```python
from build123d import *

# Parameters (mm, degrees)
F1_DEPTH  = 160
F2_R      = 2.25
F3_DEPTH  = 16.001
F4_SIZE2  = 1
F4_SIZE   = 5
F5_SIZE2  = 5
F5_SIZE   = 1
F7_DEPTH  = 5
F8_R      = 2.25
F9_DEPTH  = 2
F10_SIZE  = 1.5
F11_SIZE  = 1
F12_W     = 12
F12_H     = 6
F12_W_2   = 4
F12_H_2   = 14
F13_DEPTH = 1


# Not quite as in the source:
# - a feature names something its author has since deleted; it is built from what else it names


with BuildPart() as f1:
    # F0 (on Front) → F1 (new body)
    with BuildSketch(Plane.XZ):
        Polygon((0, 16), (0, 0), (26.5, 0), (26.5, 16), (23.5, 16), (23.5, 6), (3, 6), (3, 16), align=None)
    extrude(amount=F1_DEPTH)

    # F2 (on face) → F3 (cut, through all)
    with BuildSketch(Plane(origin=(0, 0, 0), x_dir=(1, 0, 0), z_dir=(0, 0, -1))):
        with Locations((13.25, 146)):
            Circle(F2_R)
    extrude(amount=-F3_DEPTH, mode=Mode.SUBTRACT)

    # F4
    f4_edges = [f1.edges().sort_by_distance(p)[0] for p in [
        (23.5, -80, 16),
    ]]
    f4_side = f1.faces().sort_by_distance((23.5, -80, 11))[0]
    chamfer(f4_edges, length=F4_SIZE, length2=F4_SIZE2, reference=f4_side)

    # F5
    f5_edges = [f1.edges().sort_by_distance(p)[0] for p in [
        (3, -80, 16),
    ]]
    f5_side = f1.faces().sort_by_distance((1.5, -80, 16))[0]
    chamfer(f5_edges, length=F5_SIZE, length2=F5_SIZE2, reference=f5_side)

    # F6 (on face) → F7 (cut)
    with BuildSketch(Plane(origin=(0, 0, 0), x_dir=(1, 0, 0), z_dir=(0, 0, -1))):
        Polygon((15.2707259422, 149.5), (11.2292740578, 149.5), (9.2085481157, 146), (11.2292740578, 142.5), (15.2707259422, 142.5), (17.2914518843, 146), align=None)
    extrude(amount=-F7_DEPTH, mode=Mode.SUBTRACT)

    # F8 (on face) → F9 (join)
    with BuildSketch(Plane(origin=(0, 0, 0), x_dir=(1, 0, 0), z_dir=(0, 0, -1))):
        Polygon((15.2707259422, 149.5), (11.2292740578, 149.5), (9.2085481157, 146), (11.2292740578, 142.5), (15.2707259422, 142.5), (17.2914518843, 146), align=None)
        with Locations((13.25, 146)):
            Circle(F8_R, mode=Mode.SUBTRACT)
    extrude(amount=-F9_DEPTH)

    # F10
    f10_edges = [f1.edges().sort_by_distance(p)[0] for p in [
        (11, -146, 0),
    ]]
    chamfer(f10_edges, length=F10_SIZE)

    # F11
    f11_edges = [f1.edges().sort_by_distance(p)[0] for p in [
        (0, -80, 0),
        (13.25, 0, 0),
        (26.5, -80, 0),
        (13.25, -160, 0),
        (0, 0, 8),
        (26.5, 0, 8),
        (0, -160, 8),
        (26.5, -160, 8),
        (26.5, -80, 16),
        (0, -80, 16),
    ]]
    chamfer(f11_edges, length=F11_SIZE)

    # F12 (on face) → F13 (cut)
    with BuildSketch(Plane(origin=(0, 0, 0), x_dir=(1, 0, 0), z_dir=(0, 0, -1))):
        Polygon((6.25, 18), (6.25, 10), (20.25, 10), (20.25, 18), (20.25, 32), (20.25, 33), (20.25, 40), (6.25, 40), (6.25, 33), align=None)
        with Locations((13.25, 14)):
            Rectangle(F12_W, F12_H, mode=Mode.SUBTRACT)
        with Locations((9.25, 25)):
            Rectangle(F12_W_2, F12_H_2, mode=Mode.SUBTRACT)
        Polygon((15.7156598493, 18), (12.25, 18), (12.25, 32), (19.25, 32), (19.25, 18), (16.2156598493, 18), (17.4656598493, 21), (16.4656598493, 21), (16.4656598493, 26), (15.4656598493, 26), (15.4656598493, 21), (14.4656598493, 21), align=None, mode=Mode.SUBTRACT)
        with Locations((13.25, 36)):
            Rectangle(F12_W, F12_H, mode=Mode.SUBTRACT)
    extrude(amount=-F13_DEPTH, mode=Mode.SUBTRACT)


solid = f1.part
```
Input: part model. Units: mm. Frame: model coordinates. A direction names the side the tool comes from. Give positions to 0.01 mm unless a question says otherwise; leave off trailing zeros. Order: outer loops, then holes, each group sorted by start corner. A loop starts at its lowest first (then second) coordinate and runs counter-clockwise, first axis right, second up.
1. Reachability of faces 1 (the flat face through (9, -25, 0)), 2 (the flat face through (24, -78.9, 13.5)), 3 (the flat face through (10.23, -147.77, 3.48)) from +Z, -Z, +X, -X, +Y, -Y: full face, straight path, thin tool, end or side. Return the list, or none.
Derived:
face 1: -Z, +X, -X, +Y, -Y
face 2: +Z, +Y, -Y
face 3: none
2. Section B-B on y = -55. Return the cut outline in (x, z), and give its area (3 significant figures).
Derived:
outline: (0, 1) - (1, 0) - (25.5, 0) - (26.5, 1) - (26.5, 15) - (25.5, 16) - (24.5, 16) - (23.5, 11) - (23.5, 6) - (3, 6) - (3, 11) - (2, 16) - (1, 16) - (0, 15) - close
area: 212 mm2
3. Section A-A on z = 13. Return the cut outline in (x, y).
Derived:
outline: (0, -159) - (1, -160) - (2.6, -160) - (2.6, 0) - (1, 0) - (0, -1) - close; (23.9, -160) - (25.5, -160) - (26.5, -159) - (26.5, -1) - (25.5, 0) - (23.9, 0) - close
4. Material intervals for L1, parallel to Y at x = 13.25, z = 5.45; L2, parallel to X at y = -146, z = 1.6; L3, parallel to Z at x = 6.25, y = -133, sorted ascending.
Derived:
L1: y = -160 to -148.25, -143.75 to 0
L2: x = 0 to 11, 15.5 to 26.5
L3: z = 0 to 6
5. Pin query (flat end, axial travel): pin 1 (0.5 mm diameter, centred on y = -37.5, z = 0.5, fed in from +X); pin 2 (3.5 mm diameter, centred on x = 11.5, y = -145.5, fed in from -Z); pin 3 (6 mm diameter, centred on x = 13.25, y = -146, fed in from -Z). Return the tip coordinate at first contact, or that it passes through.
Derived:
pin 1: stops at x = 26.25
pin 2: stops at z = 0.18
pin 3: stops at z = 0.75
6. Mould query, pull axis Z, two halves, no side actions, for faces 4 (the flat face through (13, -81, 0)), 5 (the flat face through (13, -142.5, 3)), 6 (the flat face through (13, -79, 6)), 7 (the flat face through (0, -79, 8)). Classes: released by +Z, released by -Z, zero draft, split by the parting line, or undercut.
Derived:
face 4: released by -Z
face 5: undercut
face 6: released by +Z
face 7: zero draft
